Input: part model. Units: mm. Frame: model coordinates. A direction names the side the tool comes from. Round coordinates to 2 decimals unless told otherwise and drop trailing zeros. Loops run counter-clockwise (first coordinate to the right, second up) from the corner with the lowest first, then second, coordinate; pieces in that order, holes last. Notation, with made-up numbers: (36, 86) -> (65, 86) arc R13 cw to (65, 91) -> close; hole circle Ø9 at (59, 44). An arc over 180 degrees is marked (long way). One line per question, with ' | ' between items. Start each with the question number.
Q1. Mould query, pull axis Z, two halves, no side actions, for faces 1 (the face through (0, 4, 38)), 2 (the face through (4.93, 14.922, 37.475)), 3 (the face through (5.07, 13.2, 1.93)). Classes: pulls with the +Z half, pulls with the -Z half, needs draft (parallel to the pull), parting line crosses it, or undercut.
Q2. Material intervals for L1, parallel to Y at x = 10.75, z = 8; L2, parallel to Y at x = 1.75, z = 69.5; L3, parallel to X at y = 7.5, z = 59, sorted ascending.
Q3. Contact query for flat-ended pins moving along their axis: P1, Ø2, axis at x = 13, z = 38, coming from the +Y side; P2, Ø6.5, axis at y = 10.5, z = 29.5, coming from the -X side; P3, Ø6, axis at x = 3, y = 17.5, coming from the -Z side. Output: stop coordinate, or through.
Q4. Cut plane A-A on x = 2.25. Return loops of the section in (y, z).
Q5. Cut plane B-B on x = 11.5. State how many separate pieces and enclosed holes the cut face has, and give its area (3 significant figures).
Q6. Access query for faces 4 (the face through (13.5, 18.45, 36.91)), 5 (the face through (5, 5, 44)). Directions: +Z, -Z, +X, -X, +Y, -Y. A direction counts if a zero-diameter tool reaches every point of the face in a straight line with its end or side. Return the directions, or none.
from build123d import *

# Parameters (mm, degrees)
ESQUISSE1_R             = 3.1
BOSS_EXTRU_1_DEPTH      = 15
CONG_1_R                = 8
CONG_2_R                = 5
ENL_V_MAT_EXTRU_1_DEPTH = 10


with BuildPart() as part:
    # Esquisse1 → Boss.-Extru.1 (new body)
    with BuildSketch(Plane(origin=(0, 0, 0), x_dir=(0, 0, -1), z_dir=(1, 0, 0))):
        Polygon((0, 0), (-76.372261843, 0), (-76.372261843, 25.120178971), (0, 15), align=None)
        with Locations((-68.372261843, 16)):
            Circle(ESQUISSE1_R, mode=Mode.SUBTRACT)
        with Locations((-8, 8)):
            Circle(ESQUISSE1_R, mode=Mode.SUBTRACT)
    extrude(amount=BOSS_EXTRU_1_DEPTH)

    # Congé1
    cong_1_edges = [part.edges().sort_by_distance(p)[0] for p in [
        (7.5, 25.120178971, 76.372261843),
        (7.5, 15, 0),
    ]]
    fillet(cong_1_edges, radius=CONG_1_R)

    # Congé2
    cong_2_edges = [part.edges().sort_by_distance(p)[0] for p in [
        (15, 3.995079138, 0),
        (15, 7.995079138, 76.372261843),
        (15, 19.920833067, 37.135227801),
    ]]
    fillet(cong_2_edges, radius=CONG_2_R)

    # Esquisse2 → Enlèv. mat.-Extru.1 (cut)
    with BuildSketch(Plane.ZY):
        with BuildLine():
            ThreePointArc((60.51684394, 17.97545174), (63.038081045, 9.904385575), (71.372261843, 8.476038278))
            Line((71.372261843, 8.476038278), (71.372261843, 5))
            Line((71.372261843, 5), (15.523961722, 5))
            ThreePointArc((15.523961722, 5), (16.082776909, 8.52793697), (15.069803831, 11.953210568))
            Line((15.069803831, 11.953210568), (60.51684394, 17.97545174))
        make_face()
    extrude(amount=-ENL_V_MAT_EXTRU_1_DEPTH, mode=Mode.SUBTRACT)


solid = part.part
Results:
1) face 1: needs draft | face 2: undercut | face 3: pulls with the -Z half
2) L1: 0 to 4.9, 11.1 to 16 | L2: 0 to 5, 7.98 to 13.11, 18.89 to 23.91 | L3: 10 to 15
3) P1: y = 19.63 | P2: x = 10 | P3: z = 3.35
4) outline: (0, 0) -> (7.99, 0) arc R8 ccw to (15.92, 6.95) -> (23.92, 67.32) arc R8 ccw to (15.99, 76.37) -> (0, 76.37) -> close; hole circle Ø6.2 at (8, 8); hole (5, 15.52) arc R8.1 cw to (11.95, 15.07) -> (17.98, 60.52) arc R8.1 cw to (8.48, 71.37) -> (5, 71.37) -> close; hole circle Ø6.2 at (16, 68.37)
5) separate pieces: 1 | enclosed holes: 2 | area: 1,420 mm^2
6) face 4: -Z, +X, +Y | face 5: -X
